Geometry: final body of the model. Coordinates: model frame, mm. A direction names the side the tool comes from. Round coordinates to 2 decimals unless told otherwise and drop trailing zeros. Loops run counter-clockwise (first coordinate to the right, second up) from the corner with the lowest first, then second, coordinate; pieces in that order, holes last. Notation, with made-up numbers: M 23,59.25 L 70,59.25 A12 cw 70,65.25 Z; hole C 11.25,-30 d2. An arc over 180 degrees is marked long. Answer as a JSON object with one key per item and string values.
```python
from build123d import *

# Parameters (mm, degrees)
F1_DEPTH = 5
F2_R     = 1.5
F3_DEPTH = 25
F4_R     = 6.5
F5_DEPTH = 25
F6_R     = 2


with BuildPart() as f1:
    # F0 (on Front) → F1 (new body)
    with BuildSketch(Plane.XZ):
        with BuildLine():
            Line((0, 14), (0, 0))
            Line((0, 0), (40, 0))
            Line((40, 0), (40, 14))
            ThreePointArc((40, 14), (43, 17), (40, 20))
            Line((40, 20), (40, 30))
            ThreePointArc((40, 30), (38.535534, 33.535534), (35, 35))
            Line((35, 35), (5, 35))
            ThreePointArc((5, 35), (1.464466, 33.535534), (0, 30))
            Line((0, 30), (0, 20))
            ThreePointArc((0, 20), (-3, 17), (0, 14))
        make_face()
    extrude(amount=F1_DEPTH)

    # F2 (on face) → F3 (cut)
    with BuildSketch(Plane.XZ.offset(5)):
        with Locations((0, 17)):
            Circle(F2_R)
        with Locations((40, 17)):
            Circle(F2_R)
    extrude(amount=-F3_DEPTH, mode=Mode.SUBTRACT)

    # F4 (on face) → F5 (cut)
    with BuildSketch(Plane.XZ.offset(5)):
        with Locations((20, 16.952448)):
            Circle(F4_R)
    extrude(amount=-F5_DEPTH, mode=Mode.SUBTRACT)

    # F6
    f6_edges = [f1.edges().sort_by_distance(p)[0] for p in [
        (0, -5, 25),
        (40, -5, 7),
        (20, -5, 0),
        (0, -5, 7),
    ]]
    fillet(f6_edges, radius=F6_R)


solid = f1.part
```
1) Cut plane A-A on z = 21.5. Return the cut outline in (x, y), and give its area (3 significant figures).
Geometry results:
{"outline": "M 0,-3 A2 ccw 2,-5 L 15.36,-5 L 15.36,0 L 0,0 Z; M 24.64,-5 L 38,-5 A2 ccw 40,-3 L 40,0 L 24.64,0 Z", "area": "152 mm2"}
2) First-contact query: pin 1 (2.5 mm diameter, centred on y = -1.5, z = 5, fed in from -X); pin 2 (2 mm diameter, centred on x = 5, y = -4.5, fed in from -Z); pin 3 (1.5 mm diameter, centred on y = -1, z = 24, fed in from +X). Flat tips, straight axial feed; report the tip coordinate or a pass-through.
Geometry results:
{"pin 1": "x = 0", "pin 2": "z = 0.06", "pin 3": "x = 40"}
3) Cut plane B-B on y = -1.9. Return the cut outline in (x, z).
Geometry results:
{"outline": "M 0,0 L 40,0 L 40,14 A3 ccw 40,20 L 40,30 A5 ccw 35,35 L 5,35 A5 ccw 0,30 L 0,20 A3 ccw 0,14 Z; hole C 0,17 d3; hole C 20,16.95 d13; hole C 40,17 d3"}
4) Set-up query: faces 1 (the face through (40, -1, 25)), 2 (the face through (0, -1, 25)), 3 (the face through (40, -1, 7)). Return all of +Z, -Z, +X, -X, +Y, -Y with unobstructed straight access to the full face (end or side cutting, diameter ignored); none if empty.
Geometry results:
{"face 1": "+Z, +X, +Y, -Y", "face 2": "+Z, -X, +Y, -Y", "face 3": "-Z, +X, +Y, -Y"}
5) Pull-direction query (X, two-part tool) for faces 4 (the face through (0, -1, 7)), 5 (the face through (14.84, -2.54, 13)), 6 (the face through (-0.195, -2.535, 18.487)), 7 (the face through (14.6, -5, 21.2)); classes: +X half, -X half, draft (parallel to the pull), parting line (faces both ways), or undercut.
Geometry results:
{"face 4": "-X half", "face 5": "undercut", "face 6": "undercut", "face 7": "draft"}
6) Cut plane C-C on z = 3. Return the cut outline in (x, y), and give its area (3 significant figures).
Geometry results:
{"outline": "M 0,-3 A2 ccw 2,-5 L 38,-5 A2 ccw 40,-3 L 40,0 L 0,0 Z", "area": "198 mm2"}
7) Line query: probe 1 along Z at (x, y) = (20, -1.65); probe 2 along X at (y, z) = (-3.3, 16); probe 3 along X at (y, z) = (-0.25, 25). Output: solid intervals per line, ascending.
Geometry results:
{"probe 1": "0 to 10.45, 23.45 to 35", "probe 2": "-2.83 to -1.12, 1.12 to 13.57, 26.43 to 38.88, 41.12 to 42.83", "probe 3": "0 to 40"}
